from build123d import *

# Parameters (mm, degrees)
SKIZZE1_W                       = 70
SKIZZE1_H                       = 25
AUFSATZ_LINEAR_AUSTRAGEN1_DEPTH = 50
SCHNITT_LINEAR_AUSTRAGEN1_DEPTH = 50
SKIZZE3_R                       = 4
SCHNITT_LINEAR_AUSTRAGEN2_DEPTH = 63.299678972


with BuildPart() as part:
    # Skizze1 → Aufsatz-Linear austragen1 (new body)
    with BuildSketch(Plane(origin=(0, 0, 0), x_dir=(1, 0, 0), z_dir=(0, 1, 0))):
        Rectangle(SKIZZE1_W, SKIZZE1_H)
    extrude(amount=AUFSATZ_LINEAR_AUSTRAGEN1_DEPTH)

    # Skizze2 → Schnitt-Linear austragen1 (cut)
    with BuildSketch(Plane.XY.offset(12.5)):
        with BuildLine():
            ThreePointArc((18.5, 25), (1.252876405, 43.457526939), (-18.33030278, 27.5))
            Line((-18.33030278, 27.5), (0, 27.5))
            Line((0, 27.5), (0, 22.5))
            Line((0, 22.5), (-18.33030278, 22.5))
            ThreePointArc((-18.33030278, 22.5), (1.252876405, 6.542473061), (18.5, 25))
        make_face()
        with BuildLine():
            Line((0, 27.5), (-18.33030278, 27.5))
            ThreePointArc((-18.33030278, 27.5), (-18.5, 25), (-18.33030278, 22.5))
            Line((-18.33030278, 22.5), (0, 22.5))
            Line((0, 22.5), (0, 27.5))
        make_face()
        with BuildLine():
            Line((-18.33030278, 27.5), (-35, 27.5))
            Line((-35, 27.5), (-35, 22.5))
            Line((-35, 22.5), (-18.33030278, 22.5))
            ThreePointArc((-18.33030278, 22.5), (-18.5, 25), (-18.33030278, 27.5))
        make_face()
    extrude(amount=-SCHNITT_LINEAR_AUSTRAGEN1_DEPTH, mode=Mode.SUBTRACT)

    # Skizze3 → Schnitt-Linear austragen2 (cut, through all)
    with BuildSketch(Plane.XZ):
        with Locations(Location((-25, 0, 0), (0, 0, 270))):
            Circle(SKIZZE3_R)
        with Locations(Location((25, 0, 0), (0, 0, 270))):
            Circle(SKIZZE3_R)
    extrude(amount=-SCHNITT_LINEAR_AUSTRAGEN2_DEPTH, mode=Mode.SUBTRACT)


solid = part.part
Verification items for the finished model (mm, model axes). A direction names the side the tool comes from. Give positions to 0.01 mm unless a question says otherwise; leave off trailing zeros. Write each loop counter-clockwise with the first axis right and the second up, starting at its lowest first coordinate (ties: lowest second). Pieces come first, ordered by that corner, then holes. Notation, with made-up numbers: M -12.75,-15 L 13.25,-15 A10 cw 13.25,-5 Z; hole C 16.25,11.25 d11. An arc over 180 degrees is marked long. Put each result on its own line as item: value. Start each with the question number.
1. Scan lines: line 1 along X through (y, z) = (28, 0); line 2 along Y through (x, z) = (-22.5, -6.5); line 3 along X through (y, z) = (31, -3.5). Record each from-to range of solid material in increasing order. Write a range as [from, to].
2. Draft check along Z on faces 1 (the face through (-35, 39, 0)), 2 (the face through (15.1, 13.5, 12.5)), 3 (the face through (-21.034, 11.092, 0.521)), 4 (the face through (28.966, 24.65, 0.521)). Enter one of: +Z half, -Z half, draft (parallel to the pull), parting line (faces both ways), or undercut.
3. Section check B-B (y = 11). Record the cut outline in (x, z).
4. Section check D-D (x = -25). Record the cut outline in (y, z), and give its area (3 significant figures).
5. Section check C-C (z = 0). Record the cut outline in (x, y).
6. Section check A-A (x = 0). Record the cut outline in (y, z), and give its area (3 significant figures).
7. Set-up check for faces 5 (the face through (-28, 27.5, 3)), 6 (the face through (-21.034, 38.592, 0.521)): record each of +Z, -Z, +X, -X, +Y, -Y from which the full face is reachable in a straight line by a thin tool's end or side.
Answer list:
1. line 1: [-35, -29], [-21, -18.26], [18.26, 21], [29, 35]
1. line 2: [0, 22.5], [27.5, 50]
1. line 3: [-35, -26.94], [-23.06, -17.5], [17.5, 23.06], [26.94, 35]
2. face 1: draft
2. face 2: +Z half
2. face 3: undercut
2. face 4: undercut
3. outline: M -35,-12.5 L -12.09,-12.5 L -12.09,12.5 L -35,12.5 Z; M 12.09,-12.5 L 35,-12.5 L 35,12.5 L 12.09,12.5 Z; hole C -25,0 d8; hole C 25,0 d8
4. outline: M 0,-12.5 L 22.5,-12.5 L 22.5,-4 L 0,-4 Z; M 0,4 L 22.5,4 L 22.5,12.5 L 0,12.5 Z; M 27.5,-12.5 L 50,-12.5 L 50,-4 L 27.5,-4 Z; M 27.5,4 L 50,4 L 50,12.5 L 27.5,12.5 Z
4. area: 765 mm2
5. outline: M -35,0 L -29,0 L -29,22.5 L -35,22.5 Z; M -35,27.5 L -29,27.5 L -29,50 L -35,50 Z; M -21,0 L 21,0 L 21,50 L -21,50 L -21,27.5 L -18.33,27.5 A18.5 cw long -18.33,22.5 L -21,22.5 Z; M 29,0 L 35,0 L 35,50 L 29,50 Z
6. outline: M 0,-12.5 L 6.5,-12.5 L 6.5,12.5 L 0,12.5 Z; M 43.5,-12.5 L 50,-12.5 L 50,12.5 L 43.5,12.5 Z
6. area: 325 mm2
7. face 5: +Z, -Z, -X
7. face 6: +Y, -Y
